CAD build for the part. Positions are in the model's coordinates, mm. Face numbers are marked on the shaded views. A direction names the side the tool comes from. Give positions to 0.01 mm unless a question says otherwise; leave off trailing zeros. Order: outer loops, then holes, each group sorted by start corner. A loop starts at its lowest first (then second) coordinate and runs counter-clockwise, first axis right, second up.
from build123d import *

# Parameters (mm, degrees)
EXTRUDE1_DEPTH     = 6.6
SKETCH2_R          = 7.1
EXTRUDE2_DEPTH     = 0.99
SKETCH15_OUTSIDE_W = 43.29
SKETCH15_OUTSIDE_H = 43.29
SKETCH15_OUTSIDE_R = 5
CUT_EXTRUDE5_DEPTH = 6.6
CUT_EXTRUDE5_DRAFT = -60
SKETCH5_W          = 30
SKETCH5_H          = 3
CHAMFER1_SIZE      = 0.75
SKETCH11_R         = 7.1
EXTRUDE3_DEPTH     = 3.3
EXTRUDE3_TAPER     = 60
FILLET1_R          = 0.495


with BuildPart() as part:
    # Sketch1 → Extrude1 (new body)
    with BuildSketch(Plane.XY):
        Polygon((5, -2.886751346), (5, 2.886751346), (0, 5.773502692), (-5, 2.886751346), (-5, -2.886751346), (0, -5.773502692), align=None)
    extrude(amount=EXTRUDE1_DEPTH)

    # Sketch2 → Extrude2 (add)
    with BuildSketch(Plane(origin=(0, 0, 0), x_dir=(-1, 0, 0), z_dir=(0, 0, -1))):
        Circle(SKETCH2_R)
    extrude(amount=-EXTRUDE2_DEPTH)


with BuildPart() as cut_extrude5_tool:
    # Sketch15 outside → Cut-Extrude5 (with draft: the straight prism first)
    with BuildSketch(Plane.XY.offset(6.6)):
        Rectangle(SKETCH15_OUTSIDE_W, SKETCH15_OUTSIDE_H)
        Circle(SKETCH15_OUTSIDE_R, mode=Mode.SUBTRACT)
    extrude(amount=-CUT_EXTRUDE5_DEPTH)
    # Cut-Extrude5: the draft: its side faces are tilted about the plane it starts from
    cut_extrude5_sides = [cut_extrude5_tool.faces().sort_by_distance(p)[0] for p in [
        (0, -21.645, 3.3),
        (21.645, 0, 3.3),
        (0, 21.645, 3.3),
        (-21.645, 0, 3.3),
        (-5, 0, 3.3),
    ]]
    draft(cut_extrude5_sides, Plane.XY.offset(6.6), CUT_EXTRUDE5_DRAFT)


with BuildPart() as part_1:
    add(part.part)

    # Cut-Extrude5: cut by cut_extrude5_tool
    add(cut_extrude5_tool.part, mode=Mode.SUBTRACT)


with BuildPart() as body_2:
    # Sketch5 → Revolve1 (revolve)
    with BuildSketch(Plane(origin=(0, 0, 0), x_dir=(0, 0, -1), z_dir=(1, 0, 0)), mode=Mode.PRIVATE) as revolve1_sk:
        with Locations((15, 1.5)):
            Rectangle(SKETCH5_W, SKETCH5_H)
    revolve(revolve1_sk.sketch.rotate(Axis((0, 0, -30), (0, 0, -1)), 90), axis=Axis((0, 0, -30), (0, 0, -1)))

    # Chamfer1
    chamfer1_edges = [body_2.edges().sort_by_distance(p)[0] for p in [
        (-3, 0, -30),
    ]]
    chamfer(chamfer1_edges, length=CHAMFER1_SIZE)


with BuildPart() as part_2:
    add(part_1.part)

    # Combine1: union body 2
    add(body_2.part)

    # Sketch10 → Revolve2 (revolve)
    with BuildSketch(Plane(origin=(0, 0, 0), x_dir=(0, 0, -1), z_dir=(1, 0, 0))):
        Polygon((12, 2.350480947), (11.697124292, 3), (-0.875, 3), (-0.875, 0), (12, 0), align=None)
    revolve(axis=Axis((0, 0, 0.875), (0, 0, -1)))

    # Sketch11 → Extrude3 (add)
    with BuildSketch(Plane.XY.offset(0.99)):
        with Locations(Location((0, 0, 0), (0, 0, 180))):
            Circle(SKETCH11_R)
    extrude(amount=EXTRUDE3_DEPTH, taper=EXTRUDE3_TAPER)

    # Fillet1
    fillet1_edges = [part_2.edges().sort_by_distance(p)[0] for p in [
        (7.1, 0, 0),
        (7.1, 0, 0.99),
    ]]
    fillet(fillet1_edges, radius=FILLET1_R)


solid = part_2.part
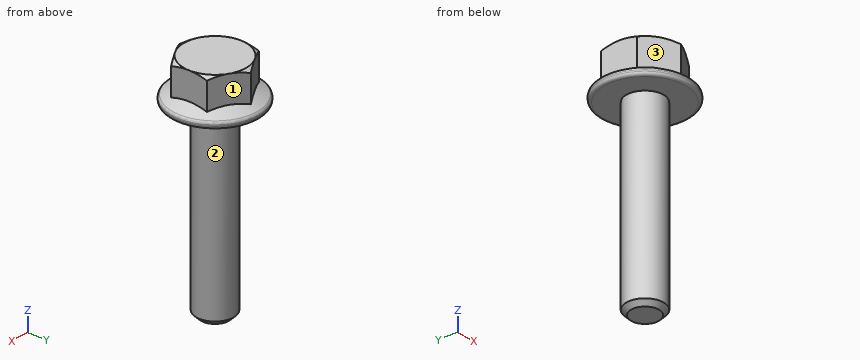
1. Pin check, flat tips, straight feed: P1, Ø2, axis at x = 0, z = -23, coming from the +Y side; P2, Ø3, axis at y = 0, z = -5, coming from the -X side; P3, Ø4, axis at x = 4, y = 2, coming from the -Z side. Stop position of each tip, or through.
2. 3-axis set-ups, long thin cutter, end or side, ignore diameter. For the marked faces 1, 2 and 3: which of +Z, -Z, +X, -X, +Y, -Y reach the whole face in a straight line?
3. Saw through at A-A on z = -26.5. Give the cut face in (x, y).
4. Wall check: line 1 (X direction, y = -1, z = 4); line 2 (Z direction, x = -1.5, y = 3.5); line 3 (Z direction, x = -4.5, y = -5.25). Give the ranges that are in metal, low to high.
Reported:
1. P1: stops at y = 3
1. P2: stops at x = -3
1. P3: stops at z = -29.78
2. face 1: +Z, +X, +Y
2. face 2: -Z
2. face 3: +Z, -X, -Y
3. outline: circle Ø6 at (0, 0)
4. line 1: x = -5 to 5
4. line 2: z = 0 to 6.6
4. line 3: z = 0.11 to 1.09
